```python
from build123d import *

# Parameters (mm, degrees)
F0_W        = 88.9
F0_H        = 165.1
F1_DEPTH    = 6.35
F2_R        = 6.34999
F3_DEPTH    = 25.4
F4_DEPTH    = 50.8
F5_C1_SIZE2 = 7.3323484187
F5_C1_SIZE  = 12.7
F5_C2_SIZE2 = 12.7
F5_C2_SIZE  = 7.3323484187
F5_C3_SIZE2 = 7.3323484187
F5_C3_SIZE  = 12.7
F5_C4_SIZE2 = 7.3323484187
F5_C4_SIZE  = 12.7
F6_C1_SIZE2 = 7.3323484187
F6_C1_SIZE  = 12.7
F6_C2_SIZE2 = 12.7
F6_C2_SIZE  = 7.3323484187
F6_C3_SIZE2 = 12.7
F6_C3_SIZE  = 7.3323484187
F6_C4_SIZE2 = 12.7
F6_C4_SIZE  = 7.3323484187


# Not quite as in the source:
# - a fillet or chamfer is up to 0.001 mm smaller than in the source, because OpenCascade refuses the exact size


with BuildPart() as f1:
    # F0 (on Top) → F1 (new body)
    with BuildSketch(Plane.XY):
        Rectangle(F0_W, F0_H)
        Polygon((-38.1, 38.1), (-38.1, 76.2), (0, 76.2), (38.1, 76.2), (38.1, -38.1), (38.1, -76.2), (0, -76.2), (-38.1, -76.2), align=None, mode=Mode.SUBTRACT)
    extrude(amount=F1_DEPTH)

    # F2 (radius 6.35 in the source; OpenCascade refuses exactly that, so slightly less here)
    f2_edges = [f1.edges().sort_by_distance(p)[0] for p in [
        (-44.45, 0, 6.35),
        (0, -82.55, 6.35),
        (44.45, 0, 6.35),
        (0, 82.55, 6.35),
    ]]
    fillet(f2_edges, radius=F2_R)

    # F0 (on Top) → F3 (join)
    with BuildSketch(Plane.XY):
        with BuildLine():
            Line((38.1, 76.2), (0, 76.2))
            Line((0, 76.2), (0, 50.8))
            ThreePointArc((0, 50.8), (-3.7197438789, 41.8197438789), (-12.7, 38.1))
            Line((-12.7, 38.1), (-38.1, 38.1))
            Line((-38.1, 38.1), (-38.1, -76.2))
            Line((-38.1, -76.2), (0, -76.2))
            Line((0, -76.2), (0, -50.8))
            ThreePointArc((0, -50.8), (3.7197438789, -41.8197438789), (12.7, -38.1))
            Line((12.7, -38.1), (38.1, -38.1))
            Line((38.1, -38.1), (38.1, 76.2))
        make_face()
    extrude(amount=F3_DEPTH)

    # F0 (on Top) → F4 (join)
    with BuildSketch(Plane.XY):
        with BuildLine():
            Line((38.1, -76.2), (38.1, -38.1))
            Line((38.1, -38.1), (12.7, -38.1))
            ThreePointArc((12.7, -38.1), (3.7197438789, -41.8197438789), (0, -50.8))
            Line((0, -50.8), (0, -76.2))
            Line((0, -76.2), (38.1, -76.2))
        make_face()
        with BuildLine():
            Line((0, 76.2), (-38.1, 76.2))
            Line((-38.1, 76.2), (-38.1, 38.1))
            Line((-38.1, 38.1), (-12.7, 38.1))
            ThreePointArc((-12.7, 38.1), (-3.7197438789, 41.8197438789), (0, 50.8))
            Line((0, 50.8), (0, 76.2))
        make_face()
    extrude(amount=F4_DEPTH)

    # F5: chamfer of 12.7 x 7.3323484187 on 4 edges, made by hand

    # F5_c1
    f5_c1_edges = [f1.edges().sort_by_distance(p)[0] for p in [
        (19.05, -76.2, 50.8),
    ]]
    f5_c1_side = f1.faces().sort_by_distance((19.05, -76.2, 50.6533530316))[0]
    chamfer(f5_c1_edges, length=F5_C1_SIZE, length2=F5_C1_SIZE2, reference=f5_c1_side)

    # F5_c2
    f5_c2_edges = [f1.edges().sort_by_distance(p)[0] for p in [
        (38.1, -53.4838257906, 50.8),
    ]]
    f5_c2_side = f1.faces().sort_by_distance((38.1, -53.4838257906, 50.6533530316))[0]
    chamfer(f5_c2_edges, length=F5_C2_SIZE, length2=F5_C2_SIZE2, reference=f5_c2_side)

    # F5_c3
    f5_c3_edges = [f1.edges().sort_by_distance(p)[0] for p in [
        (-19.05, 76.2, 50.8),
    ]]
    f5_c3_side = f1.faces().sort_by_distance((-19.05, 76.2, 50.6533530316))[0]
    chamfer(f5_c3_edges, length=F5_C3_SIZE, length2=F5_C3_SIZE2, reference=f5_c3_side)

    # F5_c4
    f5_c4_edges = [f1.edges().sort_by_distance(p)[0] for p in [
        (-38.1, 53.4838257906, 50.8),
    ]]
    f5_c4_side = f1.faces().sort_by_distance((-38.1, 53.4838257906, 50.6533530316))[0]
    chamfer(f5_c4_edges, length=F5_C4_SIZE, length2=F5_C4_SIZE2, reference=f5_c4_side)

    # F6: chamfer of 12.7 x 7.3323484187 on 4 edges, made by hand

    # F6_c1
    f6_c1_edges = [f1.edges().sort_by_distance(p)[0] for p in [
        (19.05, 76.2, 25.4),
    ]]
    f6_c1_side = f1.faces().sort_by_distance((19.05, 76.2, 25.2533530316))[0]
    chamfer(f6_c1_edges, length=F6_C1_SIZE, length2=F6_C1_SIZE2, reference=f6_c1_side)

    # F6_c2
    f6_c2_edges = [f1.edges().sort_by_distance(p)[0] for p in [
        (-38.1, -19.05, 25.4),
    ]]
    f6_c2_side = f1.faces().sort_by_distance((-37.9533530316, -19.05, 25.4))[0]
    chamfer(f6_c2_edges, length=F6_C2_SIZE, length2=F6_C2_SIZE2, reference=f6_c2_side)

    # F6_c3
    f6_c3_edges = [f1.edges().sort_by_distance(p)[0] for p in [
        (38.1, 15.3838257906, 25.4),
    ]]
    f6_c3_side = f1.faces().sort_by_distance((37.9533530316, 15.3838257906, 25.4))[0]
    chamfer(f6_c3_edges, length=F6_C3_SIZE, length2=F6_C3_SIZE2, reference=f6_c3_side)

    # F6_c4
    f6_c4_edges = [f1.edges().sort_by_distance(p)[0] for p in [
        (-15.3838257906, -76.2, 25.4),
    ]]
    f6_c4_side = f1.faces().sort_by_distance((-15.3838257906, -76.0533530316, 25.4))[0]
    chamfer(f6_c4_edges, length=F6_C4_SIZE, length2=F6_C4_SIZE2, reference=f6_c4_side)


solid = f1.part
```
Model file for the job. Use its own axes, mm. A direction names the side the tool comes from. Coordinates: 2 decimals unless noted, no trailing zeros. Loops run counter-clockwise (first coordinate to the right, second up) from the corner with the lowest first, then second, coordinate; pieces in that order, holes last. Notation, with made-up numbers: M -27.75,85.5 L 22.25,85.5 A6 cw 22.25,89.5 Z; hole C -9,15 d1. An arc over 180 degrees is marked long. Use CSV: the item, a comma, the result in double quotes. Start each with the question number.
1. Flat gauge pins, fed straight in: pin 1 (16 mm diameter, centred on y = -21, z = 17, fed in from -X); pin 2 (5 mm diameter, centred on x = 10.5, y = 50.5, fed in from +Z); pin 3 (3 mm diameter, centred on y = -9.5, z = 5.5, fed in from -X). Where does each tip first touch, or does it go through?
2. Probe probe 1 along Z at (x, y) = (3.5, 44); probe 2 along Y at (x, z) = (28, 32); probe 3 along Y at (x, z) = (-9.5, 18.5). List the from-to ranges inside material, lowest first. Write a range as [from, to].
3. Tool access for faces 1 (the flat face through (-16, 76.2, 18)), 2 (the flat face through (19.32, 72.48, 19.14)), 3 (the flat face through (-38.1, 35, 11)), 4 (the flat face through (38.1, -35, 12)): list every direction of +Z, -Z, +X, -X, +Y, -Y with a clear straight run to the whole face (end or side of a thin tool).
4. Band-saw the part on A-A, the plane z = 34. List the corners of the cut face in (x, y).
5. Band-saw the part on D-D, the plane z = 48. List the corners of the cut face in (x, y).
Entries:
1,pin 1,"stops at x = -38.1"
1,pin 2,"stops at z = 25.4"
1,pin 3,"stops at x = -43.03"
2,probe 1,"z = [0, 25.4]"
2,probe 2,"y = [-76.2, -38.1]"
2,probe 3,"y = [-72.85, 76.2]"
3,face 1,"+Z, +X, -X, +Y"
3,face 2,"+Z, +X, +Y"
3,face 3,"+Z, -X, +Y, -Y"
3,face 4,"+Z, +X, +Y, -Y"
4,outline,"M -38.1,38.1 L -12.7,38.1 A12.7 ccw 0,50.8 L 0,76.2 L -38.1,76.2 Z; M 0,-76.2 L 38.1,-76.2 L 38.1,-38.1 L 12.7,-38.1 A12.7 ccw 0,-50.8 Z"
5,outline,"M -32.38,38.1 L -12.7,38.1 A12.7 ccw 0,50.8 L 0,70.48 L -32.38,70.48 Z; M 0,-70.48 L 30.25,-70.48 L 30.25,-38.1 L 12.7,-38.1 A12.7 ccw 0,-50.8 Z"
